The listing builds one solid part. Answer for the finished solid, in the listing's coordinates (mm). A direction names the side the tool comes from. Coordinates: 2 decimals unless noted, no trailing zeros. Order: outer loops, then holes, each group sorted by start corner. A loop starts at its lowest first (then second) coordinate and runs counter-clockwise, first axis right, second up. Notation, with made-up numbers: (-22, 15) -> (11, 15) arc R8 cw to (11, 27) -> close; hole circle Ø2 at (67, 52.25). An arc over 180 degrees is marked (long way). Write item = value, one per line.
from build123d import *

# Parameters (mm, degrees)
SKETCH1_W           = 85
SKETCH1_H           = 15
BOSS_EXTRUDE1_DEPTH = 10
SKETCH2_W           = 15
SKETCH2_H           = 15
BOSS_EXTRUDE2_DEPTH = 10
FILLET3_R           = 2
SKETCH3_R           = 2
CUT_EXTRUDE1_DEPTH  = 48.565743976


with BuildPart() as part:
    # Sketch1 → Boss-Extrude1 (new body)
    with BuildSketch(Plane(origin=(0, 0, 0), x_dir=(0, 0, -1), z_dir=(1, 0, 0))):
        Rectangle(SKETCH1_W, SKETCH1_H)
    extrude(amount=BOSS_EXTRUDE1_DEPTH)

    # Sketch2 → Boss-Extrude2 (add)
    with BuildSketch(Plane.ZY):
        with Locations((-35, 0)):
            Rectangle(SKETCH2_W, SKETCH2_H)
        with Locations((35, 0)):
            Rectangle(SKETCH2_W, SKETCH2_H)
    extrude(amount=BOSS_EXTRUDE2_DEPTH)

    # Fillet3
    fillet3_edges = [part.edges().sort_by_distance(p)[0] for p in [
        (10, 0, 42.5),
        (0, -7.5, 0),
        (0, 7.5, 0),
        (10, -7.5, 0),
        (10, 0, -42.5),
        (0, -7.5, -42.5),
        (0, -7.5, 42.5),
        (0, 7.5, 42.5),
        (0, 7.5, -42.5),
        (10, 7.5, 0),
    ]]
    fillet(fillet3_edges, radius=FILLET3_R)

    # Sketch3 → Cut-Extrude1 (cut, through all)
    with BuildSketch(Plane.ZY.offset(10)):
        with Locations((-35, 0)):
            Circle(SKETCH3_R)
        with Locations(Location((35, 0, 0), (0, 0, 180))):
            Circle(SKETCH3_R)
    extrude(amount=-CUT_EXTRUDE1_DEPTH, mode=Mode.SUBTRACT)


solid = part.part
Q1. Section D-D, the plane x = 5 is taken. Give the vertices of the cut face in (y, z).
The answers:
outline = (-7.5, -40.5) arc R2 ccw to (-5.5, -42.5) -> (5.5, -42.5) arc R2 ccw to (7.5, -40.5) -> (7.5, 40.5) arc R2 ccw to (5.5, 42.5) -> (-5.5, 42.5) arc R2 ccw to (-7.5, 40.5) -> close; hole circle Ø4 at (0, -35); hole circle Ø4 at (0, 35)
Q2. A tool of negligible diameter and unlimited length cuts with its end or side. For faces 1 (the face through (0, 0, 0)), 2 (the face through (0.57, 6.9, -0.39)), 3 (the face through (-0.87, 6.9, -41.93)), 4 (the face through (0.6, -6.93, -0.39)), 5 (the face through (-0.87, 6.9, 41.93)), from which of +Z, -Z, +X, -X, +Y, -Y can it reach the whole face along a straight path? Write none if from no direction.
The answers:
face_1 = -X, +Y, -Y
face_2 = -X, +Y
face_3 = -Z, +X, -X, +Y
face_4 = -X, -Y
face_5 = +Z, +X, -X, +Y
Q3. Section C-C, the plane z = -35 is taken. Give the vertices of the cut face in (x, y).
The answers:
outline = (-10, -7.5) -> (8, -7.5) arc R2 ccw to (10, -5.5) -> (10, -2) -> (-10, -2) -> close; (-10, 2) -> (10, 2) -> (10, 5.5) arc R2 ccw to (8, 7.5) -> (-10, 7.5) -> close
Q4. Section B-B, the plane y = 0 is taken. Give the vertices of the cut face in (x, z).
The answers:
outline = (-10, -42.5) -> (8, -42.5) arc R2 ccw to (10, -40.5) -> (10, -37) -> (-10, -37) -> close; (-10, -33) -> (10, -33) -> (10, 33) -> (-10, 33) -> (-10, 27.5) -> (0, 27.5) -> (0, -27.5) -> (-10, -27.5) -> close; (-10, 37) -> (10, 37) -> (10, 40.5) arc R2 ccw to (8, 42.5) -> (-10, 42.5) -> close
Q5. Each of these flat-tipped pins is pushed along its axis until it touches: pin 1 Ø1 at (y, z) = (3.5, -2.5) entering from -X; pin 2 Ø3.5 at (y, z) = (0, -35) entering from -X. Where does it stop, or does it pass through?
The answers:
pin_1 = 0
pin_2 = through
Q6. Section A-A, the plane x = -3 is taken. Give the vertices of the cut face in (y, z), plus the area to 3 significant figures.
The answers:
outline = (-7.5, -40.5) arc R2 ccw to (-5.5, -42.5) -> (5.5, -42.5) arc R2 ccw to (7.5, -40.5) -> (7.5, -27.5) -> (-7.5, -27.5) -> close; (-7.5, 27.5) -> (7.5, 27.5) -> (7.5, 40.5) arc R2 ccw to (5.5, 42.5) -> (-5.5, 42.5) arc R2 ccw to (-7.5, 40.5) -> close; hole circle Ø4 at (0, -35); hole circle Ø4 at (0, 35)
area = 421 mm2
Q7. The mould has two halves that part along Y. Classify faces 6 (the face through (-5, 0, 27.5)), 7 (the face through (-0.14, 0.766, 33.153)), 8 (the face through (3, -7.5, -1)): released by +Y, released by -Y, zero draft, split by the parting line, or undercut.
The answers:
face_6 = zero draft
face_7 = undercut
face_8 = released by -Y
Q8. Find the intervals of material crossed by line 1 along Z through (x, y) = (-1.5, 3.5); line 2 along Y through (x, z) = (-2.5, 35); line 3 along Z through (x, y) = (5.5, -1.25), in increasing order.
The answers:
line_1 = -42.5 to -27.5, 27.5 to 42.5
line_2 = -7.5 to -2, 2 to 7.5
line_3 = -42.5 to -36.56, -33.44 to 33.44, 36.56 to 42.5
